The model under review builds one solid part; all positions refer to its coordinate system, in mm. A direction names the side the tool comes from. Round coordinates to 2 decimals unless told otherwise and drop trailing zeros. Write each loop counter-clockwise with the first axis right and the second up, starting at its lowest first coordinate (ties: lowest second). Pieces come first, ordered by that corner, then holes.
Item 1: Add section B-B (x = 2.35). State how many separate pieces and enclosed holes the cut face has, plus the area to 3 significant figures.
Item 2: Clearance check with flat-ended pins moving along their axes: pin 1 Ø1 at (x, z) = (1, -243.5) entering from -Y (3 decimals); pin 2 Ø1.6 at (x, z) = (2, -243.5) entering from +Y. State where each tip first meets the part, or that it passes through.
Item 3: Machinability: for faces 1 (the face through (1.57, 28.5, -103.45)), 2 (the face through (3.175, 196, -3)), which of the approach directions +Z, -Z, +X, -X, +Y, -Y give a long, thin tool a straight path to every point of the face, cutting with its end or side? Answer none if there is none.
Item 4: To check wall thickness, follow L1, parallel to Z at x = 1.35, y = 282.5 (3 decimals); L2, parallel to Z at x = 0.5, y = 162 (3 decimals); L3, parallel to Y at x = 1.75, z = 194. State the ranges of each line that lie inside material, in increasing order.
Item 5: Draft analysis for pull direction Z (two halves, no side actions). For faces 3 (the face through (1.57, 92.76, 116.59)), 4 (the face through (0, 196, -3)), state which applies: +Z half, -Z half, draft (parallel to the pull), parting line (faces both ways), or undercut.
Item 6: Add section A-A (y = 38). Give the boundary of the cut face in (x, z) (3 decimals), plus the area to 3 significant figures.
```python
from build123d import *

# Parameters (mm, degrees)
SKETCH1_W           = 488.95
SKETCH1_H           = 387.35
SKETCH1_R           = 5
SKETCH1_R_2         = 1.5
SKETCH1_W_2         = 20.5
SKETCH1_H_2         = 41
SKETCH1_W_3         = 100.522513204
SKETCH1_H_3         = 3.175
SKETCH1_R_3         = 9.525
SKETCH1_W_4         = 9.525
SKETCH1_W_5         = 22.225
BOSS_EXTRUDE1_DEPTH = 3.175
SKETCH2_W           = 3.175
SKETCH2_H           = 32.279166666
SKETCH2_H_2         = 32.279166667
CUT_EXTRUDE1_DEPTH  = 471.296707542
SKETCH3_W           = 6.35
SKETCH3_H           = 3.175
CUT_EXTRUDE2_DEPTH  = 471.296707542
SKETCH4_R           = 5
CUT_EXTRUDE3_DEPTH  = 471.296707542
SKETCH5_R           = 1.5
CUT_EXTRUDE4_DEPTH  = 471.296707542
SKETCH6_W           = 3.175
SKETCH6_H           = 6.35
SKETCH6_H_2         = 12.7
CUT_EXTRUDE5_DEPTH  = 471.296707542
CUT_EXTRUDE6_DEPTH  = 471.296707542


with BuildPart() as part:
    # Sketch1 → Boss-Extrude1 (new body)
    # profile 1 of 3: a face of its own
    with BuildSketch(Plane(origin=(0, 0, 0), x_dir=(0, 0, -1), z_dir=(1, 0, 0))):
        with Locations((0, 193.675)):
            Rectangle(SKETCH1_W, SKETCH1_H)
        with Locations((-141.027486796, 66.552)):
            Circle(SKETCH1_R, mode=Mode.SUBTRACT)
        with Locations((-77.027486796, 66.552)):
            Circle(SKETCH1_R, mode=Mode.SUBTRACT)
        with Locations((-215.115692196, 100.3947974)):
            Circle(SKETCH1_R_2, mode=Mode.SUBTRACT)
        with Locations((-204.955692196, 100.3947974)):
            Circle(SKETCH1_R_2, mode=Mode.SUBTRACT)
        with Locations((-210.035692196, 124.7947974)):
            Rectangle(SKETCH1_W_2, SKETCH1_H_2, mode=Mode.SUBTRACT)
        with Locations((-141.027486796, 130.552)):
            Circle(SKETCH1_R, mode=Mode.SUBTRACT)
        with Locations((-215.115692196, 149.1947974)):
            Circle(SKETCH1_R_2, mode=Mode.SUBTRACT)
        with Locations((-204.955692196, 149.1947974)):
            Circle(SKETCH1_R_2, mode=Mode.SUBTRACT)
        with Locations((-165.638743398, 189.1665)):
            Rectangle(SKETCH1_W_3, SKETCH1_H_3, mode=Mode.SUBTRACT)
        with Locations((-109.027486796, 98.552)):
            Circle(SKETCH1_R_3, mode=Mode.SUBTRACT)
        with Locations((-77.027486796, 130.552)):
            Circle(SKETCH1_R, mode=Mode.SUBTRACT)
        with BuildLine():
            ThreePointArc((241.3, 11.557), (104.709921611, 25.009948505), (-26.631076666, 64.851804754))
            Line((-26.631076666, 64.851804754), (-25.416056769, 67.78512227))
            ThreePointArc((-25.416056769, 67.78512227), (105.329333383, 28.12394177), (241.3, 14.732))
            Line((241.3, 14.732), (241.3, 11.557))
        make_face(mode=Mode.SUBTRACT)
        with BuildLine():
            ThreePointArc((-116.877486796, 196.079), (-118.377486796, 197.579), (-116.877486796, 199.079))
            Line((-116.877486796, 199.079), (-104.177486796, 199.079))
            ThreePointArc((-104.177486796, 199.079), (-102.677486796, 197.579), (-104.177486796, 196.079))
            Line((-104.177486796, 196.079), (-116.877486796, 196.079))
        make_face(mode=Mode.SUBTRACT)
        with BuildLine():
            Line((-79.177486758, 196.079), (-91.877486758, 196.079))
            ThreePointArc((-91.877486758, 196.079), (-93.377486758, 197.579), (-91.877486758, 199.079))
            Line((-91.877486758, 199.079), (-79.177486758, 199.079))
            ThreePointArc((-79.177486758, 199.079), (-77.677486758, 197.579), (-79.177486758, 196.079))
        make_face(mode=Mode.SUBTRACT)
    # profile 2 of 3: a face of its own
    with BuildSketch(Plane(origin=(0, 0, 0), x_dir=(0, 0, -1), z_dir=(1, 0, 0))):
        with Locations((-249.2375, 193.675)):
            Rectangle(SKETCH1_W_4, SKETCH1_H)
    # profile 3 of 3: a face of its own
    with BuildSketch(Plane(origin=(0, 0, 0), x_dir=(0, 0, -1), z_dir=(1, 0, 0))):
        with Locations((255.5875, 193.675)):
            Rectangle(SKETCH1_W_5, SKETCH1_H)
    extrude(amount=BOSS_EXTRUDE1_DEPTH)

    # Sketch2 → Cut-Extrude1 (cut, through all)
    with BuildSketch(Plane.ZY):
        with Locations((-242.8875, 48.41875)):
            Rectangle(SKETCH2_W, SKETCH2_H)
        with Locations((-242.8875, 112.977083334)):
            Rectangle(SKETCH2_W, SKETCH2_H_2)
        with Locations((-242.8875, 177.535416666)):
            Rectangle(SKETCH2_W, SKETCH2_H_2)
        with Locations((-242.8875, 306.652083334)):
            Rectangle(SKETCH2_W, SKETCH2_H_2)
        with Locations((-242.8875, 371.210416667)):
            Rectangle(SKETCH2_W, SKETCH2_H_2)
        with Locations((-242.8875, 242.09375)):
            Rectangle(SKETCH2_W, SKETCH2_H)
        with Locations((242.8875, 371.210416667)):
            Rectangle(SKETCH2_W, SKETCH2_H_2)
        with Locations((242.8875, 306.652083334)):
            Rectangle(SKETCH2_W, SKETCH2_H_2)
        with Locations((242.8875, 242.09375)):
            Rectangle(SKETCH2_W, SKETCH2_H)
        with Locations((242.8875, 177.535416666)):
            Rectangle(SKETCH2_W, SKETCH2_H_2)
        with Locations((242.8875, 112.977083334)):
            Rectangle(SKETCH2_W, SKETCH2_H_2)
        with Locations((242.8875, 48.41875)):
            Rectangle(SKETCH2_W, SKETCH2_H)
    extrude(amount=-CUT_EXTRUDE1_DEPTH, mode=Mode.SUBTRACT)

    # Sketch3 → Cut-Extrude2 (cut, through all)
    with BuildSketch(Plane.ZY):
        with BuildLine():
            Line((-258.7625, 206.375), (-258.7625, 193.675))
            ThreePointArc((-258.7625, 193.675), (-255.5875, 190.5), (-252.4125, 193.675))
            Line((-252.4125, 193.675), (-252.4125, 206.375))
            ThreePointArc((-252.4125, 206.375), (-255.5875, 214.687257914), (-258.7625, 206.375))
        make_face()
        with BuildLine():
            ThreePointArc((-258.7625, 374.65), (-257.83256403, 372.40493597), (-255.5875, 371.475))
            ThreePointArc((-255.5875, 371.475), (-253.34243597, 372.40493597), (-252.4125, 374.65))
            Line((-252.4125, 374.65), (-252.4125, 387.35))
            Line((-252.4125, 387.35), (-258.7625, 387.35))
            Line((-258.7625, 387.35), (-258.7625, 374.65))
        make_face()
        with Locations((-244.475, 13.1445)):
            Rectangle(SKETCH3_W, SKETCH3_H)
    extrude(amount=-CUT_EXTRUDE2_DEPTH, mode=Mode.SUBTRACT)

    # Sketch4 → Cut-Extrude3 (cut, through all)
    with BuildSketch(Plane.ZY):
        with Locations((210.035692196, 49.5947974)):
            Circle(SKETCH4_R)
        with Locations((44.935692196, 11.4947974)):
            Circle(SKETCH4_R)
        with Locations((210.035692196, 11.4947974)):
            Circle(SKETCH4_R)
    extrude(amount=-CUT_EXTRUDE3_DEPTH, mode=Mode.SUBTRACT)

    # Sketch5 → Cut-Extrude4 (cut, through all)
    with BuildSketch(Plane.ZY):
        with Locations((-19.05, 12.7)):
            Circle(SKETCH5_R)
        with Locations((19.05, 12.7)):
            Circle(SKETCH5_R)
    extrude(amount=-CUT_EXTRUDE4_DEPTH, mode=Mode.SUBTRACT)

    # Sketch6 → Cut-Extrude5 (cut, through all)
    with BuildSketch(Plane.ZY):
        Polygon((-244.475, 8.255), (-244.475, 1.905), (-244.475, 0), (-241.3, 0), (-241.3, 8.255), align=None)
        with Locations((-246.0625, 5.08)):
            Rectangle(SKETCH6_W, SKETCH6_H)
        with Locations((-246.0625, 285.75)):
            Rectangle(SKETCH6_W, SKETCH6_H_2)
        with Locations((246.0625, 285.75)):
            Rectangle(SKETCH6_W, SKETCH6_H_2)
        with Locations((246.0625, 15.875)):
            Rectangle(SKETCH6_W, SKETCH6_H_2)
    extrude(amount=-CUT_EXTRUDE5_DEPTH, mode=Mode.SUBTRACT)

    # Sketch7 → Cut-Extrude6 (cut, through all)
    with BuildSketch(Plane.ZY):
        Polygon((137.124709789, 98.948875), (137.124709789, 98.155125), (133.949709789, 98.155125), (133.949709789, 97.361375), (131.887486796, 98.552), (133.949709789, 99.742625), (133.949709789, 98.948875), align=None)
    extrude(amount=-CUT_EXTRUDE6_DEPTH, mode=Mode.SUBTRACT)


solid = part.part
```
Numbers:
1. separate pieces: 1
1. enclosed holes: 32
1. area: 197,000 mm2
2. pin 1: stops at y = 8.255
2. pin 2: stops at y = 355.07
3. face 1: +X, -X
3. face 2: +Z, -Z, +X, +Y, -Y
4. L1: z = -266.7 to -247.65, -244.475 to 244.475, 247.65 to 254
4. L2: z = -266.7 to -244.475, -241.3 to 241.3, 244.475 to 254
4. L3: y = 0 to 187.58, 190.75 to 387.35
5. face 3: undercut
5. face 4: draft
6. outline: (0, -266.7) - (3.175, -266.7) - (3.175, -244.475) - (0, -244.475) - close; (0, -241.3) - (3.175, -241.3) - (3.175, -62.715) - (0, -62.715) - close; (0, -50.7) - (3.175, -50.7) - (3.175, 241.3) - (0, 241.3) - close; (0, 244.475) - (3.175, 244.475) - (3.175, 254) - (0, 254) - close
6. area: 1,590 mm2
